Autodesk Inventor part; units mm, degrees
ref_plane "YZ Plane" through (0, 0, 0) normal (1, 0, 0) x (0, 1, 0)
ref_plane "XZ Plane" through (0, 0, 0) normal (0, 1, 0) x (-1, 0, 0)
ref_plane "XY Plane" through (0, 0, 0) normal (0, 0, 1) x (1, 0, 0)
sketch "Sketch1" plane through (0, 0, 0) normal (0, 1, 0) x (-1, 0, 0)
  circle A0 centre (0, 0) radius 1.15
  dimension "d0" = 2.3
extrude "Extrusion1" add sketch "Sketch1" along normal blind 16
sketch "Sketch2" plane through (0, 0, 0) normal (1, 0, 0) x (0, 1, 0)
  line L0 (16, -1.15) -> (16, 1.15)
  line L1 (15.5, 1.25) -> (15.5, 0)
  line L2 (16, 0) -> (15.5, 0)
  line L3 (15.5, 0) -> (13.7557, 0)
  line L4 (15.5, 1.25) -> (18, 1.25)
  line L5 (18, 1.25) -> (18, 0)
  line L6 (16, 1.15) -> (16, -1.15)
  line L7 (15.5, -1.25) -> (15.5, 0)
  line L8 (15.5, -1.25) -> (18, -1.25)
  line L9 (18, -1.25) -> (18, 0)
  point P0 (0, 0)
  dimension "d3" = 0.5
  dimension "d4" = 1.25
  dimension "d7" = 2.5
revolve "Revolution1" add sketch "Sketch2" angle 360 about axis through (0, 18, 1.25) along (0, 0, -1)
sketch "Sketch3" plane through (0, 18, 1.25) normal (0, 0, 1) x (1, 0, 0)
  circle A0 centre (0, 0) radius 2.5
  circle A1 centre (0, 0) radius 2
  point P0 (0, -18)
  dimension "d9" = 4
extrude "Extrusion2" add sketch "Sketch3" along normal blind 3.2 contours A1
sketch "Sketch4" plane through (0, 18, -1.25) normal (0, 0, -1) x (-1, 0, 0)
  circle A0 centre (0, 0) radius 2
  point P0 (0, -18)
extrude "Extrusion3" cut sketch "Sketch4" against normal blind 1.6
sketch "Sketch5" plane through (0, 0, 0) normal (1, 0, 0) x (0, 1, 0)
  line L0 (0.5, 0) -> (0.5, -1.25)
  line L1 (0, 1.15) -> (0, -1.15)
  line L2 (0, 0) -> (0.5, 0)
  line L3 (0.5, 0) -> (1.4582, 0)
  line L4 (0.5, 0) -> (0.5, -1.25)
  line L5 (-2, 0) -> (-2, -1.25)
  line L6 (0.5, -1.25) -> (-2, -1.25)
  line L7 (0.5, 0) -> (0.5, 1.25)
  line L8 (0, -1.15) -> (0, 1.15)
  line L9 (0.5, 0) -> (0.5, 1.25)
  line L10 (-2, 0) -> (-2, 1.25)
  line L11 (0.5, 1.25) -> (-2, 1.25)
  dimension "d14" = 0.5
  dimension "d15" = 1.25
  dimension "d16" = 2.5
revolve "Revolution2" add sketch "Sketch5" angle 360 about axis through (0, -2, 0) along (0, 0, 1)
sketch "Sketch6" plane through (0, -2, 1.25) normal (0, 0, 1) x (1, 0, 0)
  circle A0 centre (0, 0) radius 2.5
  circle A1 centre (0, 0) radius 1.5
  point P0 (0, 2)
  dimension "d18" = 3
extrude "Extrusion4" add sketch "Sketch6" along normal blind 5.7 contours A1
sketch "Sketch7" plane through (0, -2, -1.25) normal (0, 0, -1) x (-1, 0, 0)
  circle A0 centre (0, 0) radius 1.5
  point P0 (0, 2)
extrude "Extrusion5" cut sketch "Sketch7" against normal blind 0.5
properties part number "101-03" material "Aluminum 6061"
Here's how the part is built. I have some questions about the finished solid (model axes, mm). A direction names the side the tool comes from. Round coordinates to 2 decimals unless told otherwise and drop trailing zeros. Write each loop counter-clockwise with the first axis right and the second up, starting at its lowest first coordinate (ties: lowest second). Pieces come first, ordered by that corner, then holes.
Q1. Will these pins go through, and if not, where does the flat tip stop? P1, Ø1.5, axis at x = -0.5, y = -2, coming from the -Z side; P2, Ø3, axis at x = 1, y = 1, coming from the +Z side; P3, Ø2, axis at x = 0.5, y = 18, coming from the +Z side.
Q2. If we section it at B-B on y = -2: Write out the boundary of the cut face in (x, z).
Q3. Which directions (+Z, -Z, +X, -X, +Y, -Y) give clear straight access to the entire face, cutting with the end or side of a thin tool? Please do faces 3 (the flat face through (2, -2, -1.25)), 4 (the flat face through (0, 18, 4.45)), 5 (the flat face through (0, -2, -0.75)), 6 (the flat face through (2, -2, 1.25)).
Q4. Please list where these lines run through material, in increasing order: probe 1 along Y at (x, z) = (0, -0.9); probe 2 along Y at (x, z) = (-0.05, 3.5); probe 3 along Z at (x, y) = (-0.05, 19).
Q5. If we section it at D-D on z = 3.25: Write out the boundary of the cut face in (x, y).
Q6. If we mould it in two halves opening along Y, with no side actions, what happens to faces 1 (the flat face through (0, -2, 6.95)), 2 (the cylindrical face through (0.91, 7.89, 0.7))? For each: +Y half, -Y half, draft (parallel to the pull), parting line (faces both ways), or undercut.
Q7. If we section it at A-A on z = 0: Write out the boundary of the cut face in (x, y), plus the area to 3 significant figures.
Q8. If we section it at C-C on x = 0: Write out the boundary of the cut face in (y, z).
Answer below:
1. P1: stops at z = -0.75
1. P2: stops at z = 1.25
1. P3: stops at z = 4.45
2. outline: (-2.5, -1.25) - (-1.5, -1.25) - (-1.5, -0.75) - (1.5, -0.75) - (1.5, -1.25) - (2.5, -1.25) - (2.5, 1.25) - (1.5, 1.25) - (1.5, 6.95) - (-1.5, 6.95) - (-1.5, 1.25) - (-2.5, 1.25) - close
3. face 3: -Z, +X, -X, +Y, -Y
3. face 4: +Z, +X, -X, +Y
3. face 5: -Z
3. face 6: +Z
4. probe 1: y = -4.5 to -3.5, -0.5 to 16, 20 to 20.5
4. probe 2: y = -3.5 to -0.5, 16 to 20
4. probe 3: z = 0.35 to 4.45
5. outline: circle Ø4 at (0, 18); circle Ø3 at (0, -2)
6. face 1: draft
6. face 2: undercut
7. outline: (-1.15, 0.22) arc R2.5 ccw (long way) to (1.15, 0.22) - (1.15, 15.78) arc R2.5 ccw (long way) to (-1.15, 15.78) - close; hole circle Ø4 at (0, 18)
7. area: 61.6 mm2
8. outline: (-4.5, -1.25) - (-3.5, -1.25) - (-3.5, -0.75) - (-0.5, -0.75) - (-0.5, -1.25) - (0.5, -1.25) - (0.5, -1.15) - (15.5, -1.15) - (15.5, -1.25) - (16, -1.25) - (16, 0.35) - (20, 0.35) - (20, -1.25) - (20.5, -1.25) - (20.5, 1.25) - (20, 1.25) - (20, 4.45) - (16, 4.45) - (16, 1.25) - (15.5, 1.25) - (15.5, 1.15) - (0.5, 1.15) - (0.5, 1.25) - (-0.5, 1.25) - (-0.5, 6.95) - (-3.5, 6.95) - (-3.5, 1.25) - (-4.5, 1.25) - close
